from build123d import *

# Parameters (mm, degrees)
SKETCH_1_W          = 120
SKETCH_1_H          = 80
SKETCH_1_R          = 2.5
EXTRUDE_1_DEPTH     = 5
SKETCH_3_R          = 1.5
SKETCH_3_R_2        = 1
CUT_EXTRUDE_1_DEPTH = 10
FILLET_1_R          = 5


with BuildPart() as part:
    # 草图1 → 凸台-拉伸1 (new body)
    with BuildSketch(Plane.XY):
        Rectangle(SKETCH_1_W, SKETCH_1_H)
        with Locations((-47.5, 15)):
            Circle(SKETCH_1_R, mode=Mode.SUBTRACT)
        with Locations((47.5, 15)):
            Circle(SKETCH_1_R, mode=Mode.SUBTRACT)
        with Locations((47.5, -15)):
            Circle(SKETCH_1_R, mode=Mode.SUBTRACT)
        with Locations((-47.5, -15)):
            Circle(SKETCH_1_R, mode=Mode.SUBTRACT)
    extrude(amount=EXTRUDE_1_DEPTH)

    # 草图3 → 切除-拉伸1 (cut)
    with BuildSketch(Plane(origin=(0, 0, 0), x_dir=(-1, 0, 0), z_dir=(0, 0, -1))):
        with Locations((51.702251253, -25)):
            Circle(SKETCH_3_R)
        with Locations((1.702251253, -25)):
            Circle(SKETCH_3_R)
        with Locations((1.702251253, 25)):
            Circle(SKETCH_3_R)
        with Locations((51.702251253, 25)):
            Circle(SKETCH_3_R)
        with Locations((-8, -32.5)):
            Circle(SKETCH_3_R_2)
        with Locations((-53, -32.5)):
            Circle(SKETCH_3_R_2)
        with Locations((-53, 32.5)):
            Circle(SKETCH_3_R_2)
        with Locations((-8, 32.5)):
            Circle(SKETCH_3_R_2)
    extrude(amount=-CUT_EXTRUDE_1_DEPTH, mode=Mode.SUBTRACT)

    # 圆角1
    fillet_1_edges = [part.edges().sort_by_distance(p)[0] for p in [
        (60, -40, 2.5),
        (-60, -40, 2.5),
        (-60, 40, 2.5),
        (60, 40, 2.5),
    ]]
    fillet(fillet_1_edges, radius=FILLET_1_R)


solid = part.part
Could you check a few things on this model? Use its own coordinates, in mm. Give positions to 0.01 mm unless a question says otherwise; leave off trailing zeros. Order: outer loops, then holes, each group sorted by start corner. A loop starts at its lowest first (then second) coordinate and runs counter-clockwise, first axis right, second up. Notation, with made-up numbers: (-32.75, 36) - (-11.75, 36) arc R20 ccw to (-11.75, 54) - close; hole circle Ø11 at (19, -17.75). An arc over 180 degrees is marked (long way). One line per item, written item: value. Start each with the question number.
1. Imagine slicing it at B-B on x = -47.5. List the corners of the cut face in (y, z) for me.
2. Imagine slicing it at A-A on y = -15. List the corners of the cut face in (x, z) for me, plus the area to 3 significant figures.
3. If I drill on probe 1 along Y at (x, z) = (47.5, 2.8); probe 2 along Y at (x, z) = (47, 3.1); probe 3 along X at (y, z) = (16, 3.75), over which ranges is the centre line in solid material (lowest first)?
4. Thinking about a two-plate mould opening in X: for faces 1 (the face through (-1, 40, 2)), 2 (the face through (-53.133, -24.549, 2.465)), 3 (the face through (58, 39, 3)), which applies, +X half, -X half, draft (parallel to the pull), parting line (faces both ways), or undercut?
Values:
1. outline: (-40, 0) - (-17.5, 0) - (-17.5, 5) - (-40, 5) - close; (-12.5, 0) - (12.5, 0) - (12.5, 5) - (-12.5, 5) - close; (17.5, 0) - (40, 0) - (40, 5) - (17.5, 5) - close
2. outline: (-60, 0) - (-50, 0) - (-50, 5) - (-60, 5) - close; (-45, 0) - (45, 0) - (45, 5) - (-45, 5) - close; (50, 0) - (60, 0) - (60, 5) - (50, 5) - close
2. area: 550 mm²
3. probe 1: -40 to -17.5, -12.5 to 12.5, 17.5 to 40
3. probe 2: -40 to -17.45, -12.55 to 12.55, 17.45 to 40
3. probe 3: -60 to -49.79, -45.21 to 45.21, 49.79 to 60
4. face 1: draft
4. face 2: undercut
4. face 3: +X half
